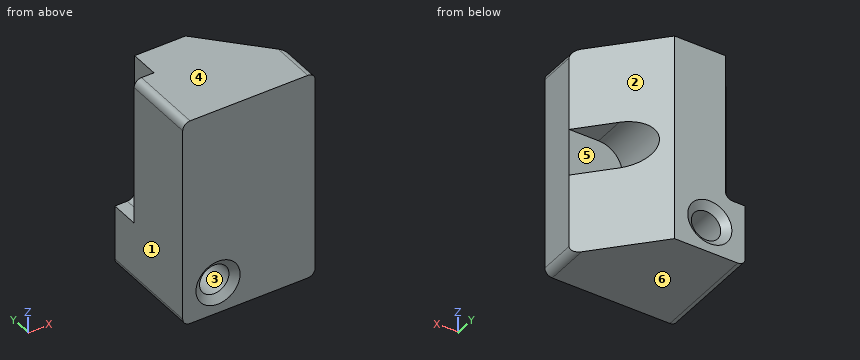
```python
from build123d import *
from OCP.BRepFilletAPI import BRepFilletAPI_MakeChamfer

# Parameters (mm, degrees)
BOSS_EXTRUDE1_DEPTH = 142
SKETCH2_W           = 13.438345352
SKETCH2_H           = 19.890532225
CUT_EXTRUDE1_DEPTH  = 100
SKETCH4_R           = 10
CUT_EXTRUDE2_DEPTH  = 100
CUT_EXTRUDE3_DEPTH  = 100
CHAMFER1_SIZE       = 5
CHAMFER1_SIZE2      = 3.906428133
FILLET5_R           = 5
FILLET6_R           = 5
FILLET7_R           = 5


with BuildPart() as part:
    # Sketch1 → Boss-Extrude1 (new body)
    with BuildSketch(Plane.XY):
        Polygon((-45, -35), (45, -35), (45, -10), (3, 35), (-45, 35), align=None)
    extrude(amount=-BOSS_EXTRUDE1_DEPTH)

    # Sketch2 → Cut-Extrude1 (cut)
    with BuildSketch(Plane.XY):
        with Locations((-38.280827324, 25.054733887)):
            Rectangle(SKETCH2_W, SKETCH2_H)
    extrude(amount=-CUT_EXTRUDE1_DEPTH, mode=Mode.SUBTRACT)

    # Sketch4 → Cut-Extrude2 (cut)
    with BuildSketch(Plane(origin=(0, 35, 0), x_dir=(1, 0, 0), z_dir=(0, 1, 0))):
        with Locations(Location((-21, 121, 0), (0, 0, 180))):
            Circle(SKETCH4_R)
    extrude(amount=-CUT_EXTRUDE2_DEPTH, mode=Mode.SUBTRACT)

    # 3DSketch2 → Cut-Extrude3 (cut)
    with BuildSketch(Plane(origin=(45, -10, -55), x_dir=(-0.5299989400031795, 0, -0.8479983040050884), z_dir=(0, 1, 0))):
        with BuildLine():
            Line((0, 0), (10.5999788, 16.95996608))
            ThreePointArc((10.5999788, 16.95996608), (32.647934704, 22.047955904), (37.735924528, 0))
            Line((37.735924528, 0), (27.135945728, -16.95996608))
            Line((27.135945728, -16.95996608), (0, 0))
        make_face()
    extrude(amount=CUT_EXTRUDE3_DEPTH, mode=Mode.SUBTRACT)

    # Chamfer1: one chamfer whose edges measure the first distance from different faces: ONE call of the kernel's chamfer builder (chamfer() names one face for all edges)
    chamfer1_edges_1 = [part.edges().sort_by_distance(p)[0] for p in [
        (-11, -35, -121),
    ]]
    chamfer1_side_1 = [part.faces().sort_by_distance(p)[0] for p in [
        (0.529233825, -35, -69.739919465),
    ]]
    chamfer1_edges_2 = [part.edges().sort_by_distance(p)[0] for p in [
        (-11, 35, -121),
    ]]
    chamfer1_side_2 = [part.faces().sort_by_distance(p)[0] for p in [
        (-16.497761799, 35, -73.425852449),
    ]]
    chamfer1 = BRepFilletAPI_MakeChamfer(part.part.solid().wrapped)
    for e in chamfer1_edges_1:
        chamfer1.Add(CHAMFER1_SIZE, CHAMFER1_SIZE2, e.wrapped, chamfer1_side_1[0].wrapped)  # the first distance lies on this face
    for e in chamfer1_edges_2:
        chamfer1.Add(CHAMFER1_SIZE, CHAMFER1_SIZE2, e.wrapped, chamfer1_side_2[0].wrapped)  # the first distance lies on this face
    add(Compound.cast(chamfer1.Shape()), mode=Mode.REPLACE)

    # Fillet5
    fillet5_edges = [part.edges().sort_by_distance(p)[0] for p in [
        (-31.561654648, 25.054733887, -100),
    ]]
    fillet(fillet5_edges, radius=FILLET5_R)

    # Fillet6
    fillet6_edges = [part.edges().sort_by_distance(p)[0] for p in [
        (-45, -9.945266113, 0),
        (45, -22.5, 0),
    ]]
    fillet(fillet6_edges, radius=FILLET6_R)

    # Fillet7
    fillet7_edges = [part.edges().sort_by_distance(p)[0] for p in [
        (-45, 0, -142),
        (45, -22.5, -142),
    ]]
    fillet(fillet7_edges, radius=FILLET7_R)


solid = part.part
```
Input: part model. Units: mm. Frame: model coordinates. Face numbers are marked on the shaded views. A direction names the side the tool comes from. Round coordinates to 2 decimals unless told otherwise and drop trailing zeros. Write each loop counter-clockwise with the first axis right and the second up, starting at its lowest first coordinate (ties: lowest second). Pieces come first, ordered by that corner, then holes. Notation, with made-up numbers: M 64,86.25 L 120,86.25 A16 ccw 120,98.25 Z; hole C -27.75,-39.5 d10. An arc over 180 degrees is marked long. Write each question's results on one line, items separated by ' | '.
Q1. Line query: line 1 along Z through (x, y) = (-21, 4); line 2 along Z through (x, y) = (20.5, 15); line 3 along Y through (x, z) = (-38, -83). Output: solid intervals per line, ascending.
Results:
line 1: z = -142 to -131, -111 to 0 | line 2: z = -142 to -86.35, -55.65 to 0 | line 3: y = -35 to 15.11
Q2. Draft query along X for the marked faces 1, 2, 3 and 4. Return one class per face: released by +X, released by -X, zero draft, split by the parting line, or undercut.
Results:
face 1: released by -X | face 2: released by +X | face 3: undercut | face 4: zero draft
Q3. Pin query (flat end, axial travel): P1, Ø16, axis at x = 25, z = -78, coming from the +Y side; P2, Ø23, axis at x = -21, z = -121, coming from the +Y side; P3, Ø9.5, axis at x = -42.5, y = 21, coming from the +Z side. Return the tip coordinate at first contact, or that it passes through.
Results:
P1: stops at y = -10 | P2: stops at y = 32.27 | P3: stops at z = -100
Q4. Section query A-A (x = -21). Return loops of the section in (y, z).
Results:
outline: M -35,-142 L 35,-142 L 35,-136 L 31.09,-131 L -31.09,-131 L -35,-136 Z; M -35,-106 L -31.09,-111 L 31.09,-111 L 35,-106 L 35,0 L -35,0 Z
Q5. Section query C-C (z = -71). Return loops of the section in (x, y), and give its area (3 significant figures).
Results:
outline: M -45,-35 L 45,-35 L 45,-10 L 9,-10 L 9,28.57 L 3,35 L -31.56,35 L -31.56,15.11 L -45,15.11 Z | area: 4,390 mm^2
Q6. Section query D-D (x = 38). Return loops of the section in (y, z), and give its area (4 significant figures).
Results:
outline: M -35,-142 L -2.5,-142 L -2.5,-87 L -10,-87 L -10,-55 L -2.5,-55 L -2.5,0 L -35,0 Z | area: 4,375 mm^2
Q7. Access query for the marked faces 5 and 6. Directions: +Z, -Z, +X, -X, +Y, -Y. A direction counts if a zero-diameter tool reaches every point of the face in a straight line with its end or side. Return the directions, or none.
Results:
face 5: +X, +Y | face 6: -Z, +X, -X, +Y, -Y
Q8. Section query B-B (y = -12.5). Return loops of the section in (x, z).
Results:
outline: M -45,-137 A5 ccw -40,-142 L 40,-142 A5 ccw 45,-137 L 45,-5 A5 ccw 40,0 L -40,0 A5 ccw -45,-5 Z; hole C -21,-121 d20
